Autodesk Inventor part; units mm, degrees
ref_plane "YZ Plane" through (0, 0, 0) normal (1, 0, 0) x (0, 1, 0)
ref_plane "XZ Plane" through (0, 0, 0) normal (0, 1, 0) x (-1, 0, 0)
ref_plane "XY Plane" through (0, 0, 0) normal (0, 0, 1) x (1, 0, 0)
sketch "Sketch1" plane through (0, 0, 0) normal (0, 1, 0) x (-1, 0, 0)
  circle A0 centre (0, 0) radius 8
  dimension "d0" = 16
extrude "Extrusion1" add sketch "Sketch1" along normal blind 13
sketch "Sketch2" plane through (0, 13, 0) normal (0, 1, 0) x (1, 0, 0)
  circle A0 centre (0, 0) radius 3
  dimension "d3" = 6
extrude "Extrusion2" add sketch "Sketch2" along normal blind 1.85
sketch "Sketch3" plane through (0, 14.85, 0) normal (0, 1, 0) x (1, 0, 0)
  circle A0 centre (0, 0) radius 1.5
  dimension "d6" = 3
extrude "Extrusion3" add sketch "Sketch3" along normal blind 8
sketch "Sketch4" plane through (0, 22.85, 0) normal (0, 1, 0) x (1, 0, 0)
  circle A0 centre (0, 0) radius 1.5
  line L0 (0.9, 0) -> (0.9, 1.2)
  line L1 (0.9, 1.2) -> (0.9, -1.2)
  circle A1 centre (0, 0) radius 3
  arc A2 (0.9, -1.2) -> (0.9, 1.2) centre (0, 0) ccw
extrude "Extrusion4" cut sketch "Sketch4" against normal blind 7 contours A0 L1 L0 picked at (0.9839, 0.7204)
sketch "Sketch5" plane through (0, 13, 0) normal (0, 1, 0) x (1, 0, 0)
  circle A0 centre (5, 0) radius 1.5
  circle A1 centre (-5, 0) radius 1.5
  point P0 (0, 0)
extrude "Extrusion5" cut sketch "Sketch5" against normal blind 2
sketch "Sketch6" plane through (0, 13, 0) normal (0, 1, 0) x (1, 0, 0)
  circle A0 centre (0, 0) radius 8
  circle A1 centre (0, -5.45) radius 0.775
  line L0 (-8, 0) -> (8, 0)
  circle A2 centre (0, 5.45) radius 0.775
extrude "Extrusion6" cut sketch "Sketch6" against normal blind 2 contours A1 | A2
sketch "Sketch7" plane through (0, 13, 0) normal (0, 1, 0) x (1, 0, 0)
  point P0 (0, 0)
sketch "Sketch8" plane through (0, 0, 0) normal (0, -1, 0) x (1, 0, 0)
  circle A0 centre (0, 0) radius 7.725
  dimension "d22" = 15.45
extrude "Extrusion7" add sketch "Sketch8" along normal blind 26.35
sketch "Sketch9" plane through (0, -26.35, 0) normal (0, -1, 0) x (1, 0, 0)
  line L0 (0, -6) -> (-4.8658, -6)
  circle A0 centre (0, 0) radius 7.725
  line L1 (0, -6) -> (4.8658, -6)
  line L2 (0, 6) -> (-4.8653, 6.0004)
  line L3 (0, 6) -> (4.8652, 6.0004)
  arc A1 (-4.8658, -6) -> (4.8658, -6) centre (0, 0) ccw
  arc A2 (4.8652, 6.0004) -> (-4.8653, 6.0004) centre (0, 0) ccw
extrude "Extrusion8" cut sketch "Sketch9" against normal blind 26.35 contours L1 A0 L0 | A0 L3 L2
sketch "Sketch10" plane through (0, -26.35, 0) normal (0, -1, 0) x (1, 0, 0)
  circle A0 centre (0, 0) radius 2.325
  dimension "d29" = 4.65
extrude "Extrusion9" add sketch "Sketch10" along normal blind 2.4
fillet "Fillet1" radius 0.125 1 edges at (-2.325, -28.75, 0)
fillet "Fillet2" radius 0.05 1 edges at (-3, 14.85, 0)
fillet "Fillet3" radius 0.25 3 edges at (4.8658, -13.175, -6) (-4.8653, -13.175, 6.0004) (4.8652, -13.175, 6.0004)
properties part number "Motor DC 21mm"
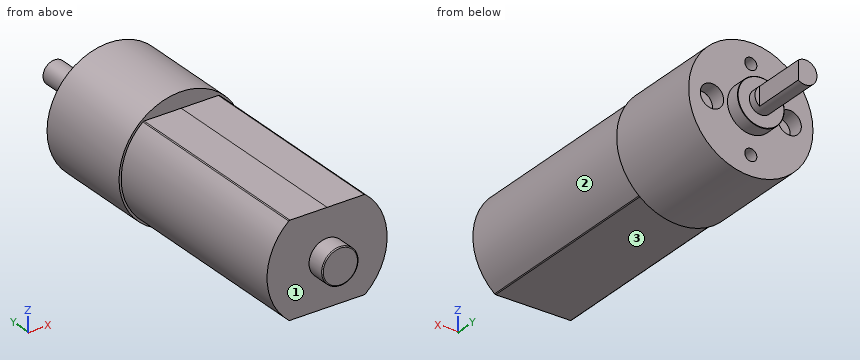
Design review of the part built by this model. Coordinates are the model's own, in mm. Face numbers are marked on the shaded views. A direction names the side the tool comes from. Coordinates: 2 decimals unless noted, no trailing zeros. Loops run counter-clockwise (first coordinate to the right, second up) from the corner with the lowest first, then second, coordinate; pieces in that order, holes last. Notation, with made-up numbers: (-28, 36) - (-2, 36) arc R27 ccw to (-2, 56) - close; hole circle Ø5 at (79, 85). An arc over 180 degrees is marked (long way). Use CSV: the item, a comma, the result in double quotes. Start each with the question number.
1) Wall thickness on L1, parallel to Z at x = 0, y = 12.3 (3 decimals); L2, parallel to Y at x = 3.25, z = -5.5; L3, parallel to Z at x = -4, y = -3: over which ranges is each line inside the solid? List them lowest first. Write a range as from..to.
2) Tool access review of the marked faces 1, 2 and 3: name each direction out of +Z, -Z, +X, -X, +Y, -Y from which nothing blocks a thin tool from reaching the whole face with its end or side.
3) For pin 1 Ø1.2 at (x, z) = (0, -5) entering from +Y; pin 2 Ø4 at (x, y) = (1, -7) entering from +Z; pin 3 Ø1.2 at (x, z) = (0, -5.45) entering from +Y, all flat-tipped, find the tip position at first contact; note any pin that passes through.
4) Consider section D-D on z = 4. Write out the cut boundary in (x, y).
5) Consider section B-B on y = 1. Write out the cut boundary in (x, z).
6) Consider section C-C on x = 5.5. Write out the cut boundary in (y, z).
Geometry says:
1,L1,"-8..-6.225, -4.675..4.675, 6.225..8"
1,L2,"-26.35..13"
1,L3,"-6..6"
2,face 1,"-Y"
2,face 2,"+X, -Y"
2,face 3,"-Z, +X, -X, -Y"
3,pin 1,"y = 13"
3,pin 2,"z = 6"
3,pin 3,"y = 11"
4,outline,"(-6.93, 0) - (-6.61, 0) - (-6.61, -26.35) - (6.61, -26.35) - (6.61, 0) - (6.93, 0) - (6.93, 13) - (-6.93, 13) - close"
5,outline,"circle Ø16 at (0, 0)"
6,outline,"(-26.35, -5.42) - (0, -5.42) - (0, -5.81) - (13, -5.81) - (13, -1.41) - (11, -1.41) - (11, 1.41) - (13, 1.41) - (13, 5.81) - (0, 5.81) - (0, 5.42) - (-26.35, 5.42) - close"
